Read the model definition and answer for the solid it produces. Units are mm, in the model's axes. Round coordinates to 2 decimals unless told otherwise and drop trailing zeros. Order: outer loops, then holes, each group sorted by start corner. A loop starts at its lowest first (then second) coordinate and runs counter-clockwise, first axis right, second up. Notation, with made-up numbers: M 49.25,43.5 L 79.25,43.5 A10 cw 79.25,56.5 Z; hole C 80.25,20 d6. An arc over 180 degrees is marked long. Answer as CSV lines item,"result".
```python
from build123d import *

# Parameters (mm, degrees)
F1_DEPTH = 2
F3_DEPTH = 25


with BuildPart() as f1:
    # F0 (on Front) → F1 (new body)
    with BuildSketch(Plane.XZ):
        Polygon((-48.7309247255, 48.1939427555), (-73.2373036639, 43.8981056213), (-56.2486425042, 24.2983382195), (-59.4705231488, 0), (-36.618651832, 10.8738420531), (-13.5587416589, 0), (-16.5121313184, 25.3722984344), (0, 43.6296164989), (-24.835318327, 48.1939427555), (-36.618651832, 69.941624999), align=None)
    extrude(amount=F1_DEPTH)

    # F2 (on face) → F3 (cut)
    with BuildSketch(Plane.XZ.offset(2)):
        with BuildLine():
            add(Edge.make_bspline(
                [(-42.8241454065, 42.018674314), (-42.215811031, 42.0156652147), (-40.0248783805, 42.0048278626), (-40.4838324873, 34.9711646084), (-40.8153533936, 29.8904683441)],
                knots=[0, 0, 0, 0, 0.2776600072, 1, 1, 1, 1], degree=3))
            add(Edge.make_bspline(
                [(-42.8241454065, 42.018674314), (-43.1211611971, 41.817411735), (-43.9730260473, 41.2401746918), (-44.7285981197, 37.046533313), (-45.4586501607, 30.6342959102), (-42.8138464069, 26.7380268066), (-41.4719755399, 28.85470644), (-40.8153533936, 29.8904683441)],
                knots=[0, 0, 0, 0, 0.1173333317, 0.3365213034, 0.622595536, 0.815323415, 1, 1, 1, 1], degree=3))
        make_face()
        with BuildLine():
            add(Edge.make_bspline(
                [(-30.4665230215, 41.817411735), (-30.7828157907, 42.0132867548), (-31.5566720158, 42.0016665583), (-32.758418401, 39.7526667198), (-32.4605723261, 35.8588497009), (-32.5698270564, 31.5889371812), (-32.4797926297, 29.976349033), (-31.378124697, 27.4296174444), (-27.4746603802, 28.3933105876), (-27.939027342, 38.0017634716), (-29.776947659, 41.3903688148), (-30.4665230215, 41.817411735)],
                knots=[0, 0, 0, 0, 0.0595652349, 0.1516653863, 0.2790521251, 0.4073989231, 0.4888413673, 0.5825769232, 0.6810659238, 0.8701370299, 1, 1, 1, 1], degree=3))
        make_face()
    extrude(amount=-F3_DEPTH, mode=Mode.SUBTRACT)


solid = f1.part
```
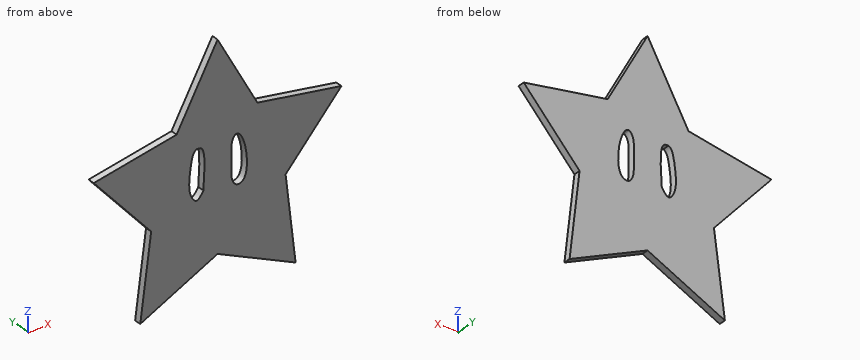
Item 1: Find the intervals of material crossed by probe 1 along X at (y, z) = (-0.45, 33); probe 2 along Z at (x, y) = (-30, -0.15); probe 3 along X at (y, z) = (-0.75, 12), in increasing order. Write a range as [from, to].
Ans:
probe 1,"[-63.79, -45.01], [-40.62, -32.53], [-27.93, -9.61]"
probe 2,"[7.75, 27.93], [41.39, 57.73]"
probe 3,"[-57.88, -14.96]"
Item 2: A cutting plane is placed at D-D, the plane x = -12. Determine the outline of the cut face in (y, z).
Ans:
outline,"M -2,30.36 L 0,30.36 L 0,45.84 L -2,45.84 Z"
Item 3: A cutting plane is placed at B-B, the plane y = -1.15. Give the number of separate pieces and of enclosed holes in the cut face, and give its area (3 significant figures).
Ans:
separate pieces,"1"
enclosed holes,"2"
area,"2,250 mm2"
Item 4: A cutting plane is placed at A-A, the plane z = 7.5. Determine the outline of the cut face in (x, y).
Ans:
outline,"M -58.48,-2 L -43.71,-2 L -43.71,0 L -58.48,0 Z; M -29.46,-2 L -14.43,-2 L -14.43,0 L -29.46,0 Z"
Item 5: A cutting plane is placed at C-C, the plane z = 20. Determine the outline of the cut face in (x, y).
Ans:
outline,"M -56.82,-2 L -15.89,-2 L -15.89,0 L -56.82,0 Z"
